Autodesk Inventor part; units mm, degrees
ref_plane "YZ Plane" through (0, 0, 0) normal (1, 0, 0) x (0, 1, 0)
ref_plane "XZ Plane" through (0, 0, 0) normal (0, 1, 0) x (-1, 0, 0)
ref_plane "XY Plane" through (0, 0, 0) normal (0, 0, 1) x (1, 0, 0)
sketch "スケッチ1" plane through (0, 0, 0) normal (0, 0, 1) x (1, 0, 0)
  line L0 (0, 0) -> (85, 0)
  line L1 (85, 0) -> (85, 42)
  line L2 (85, 42) -> (0, 42)
  line L3 (0, 42) -> (0, 0)
  dimension "d0" = 85
  dimension "d1" = 42
extrude "押し出し1" add sketch "スケッチ1" along normal blind 6
sketch "スケッチ2" plane through (0, 0, 0) normal (-1, 0, 0) x (0, 0, 1)
  circle A0 centre (3, 36) radius 1.2
  circle A1 centre (3, 6) radius 1.2
  line L0 (0, 42) -> (6, 42)
  line L1 (0, 0) -> (6, 0)
  dimension "d4" = 2.4
  dimension "d5" = 2.4
  dimension "d6" = 6
  dimension "d7" = 6
extrude "押し出し2" cut sketch "スケッチ2" against normal blind 8
sketch "スケッチ3" plane through (85, 0, 0) normal (1, 0, 0) x (0, 0, -1)
  circle A0 centre (-3, 6) radius 1.2
  circle A1 centre (-3, 6) radius 1.2
  circle A2 centre (-3, 36) radius 1.2
  circle A3 centre (-3, 36) radius 1.2
  point P0 (0, 0)
extrude "押し出し3" cut sketch "スケッチ3" against normal blind 8
sketch "スケッチ4" plane through (0, 0, 6) normal (0, 0, 1) x (1, 0, 0)
  line L0 (0, 0) -> (85, 0)
  line L1 (85, 0) -> (85, 42)
  line L2 (85, 42) -> (0, 42)
  line L3 (0, 42) -> (0, 0)
  line L4 (13.6951, 28.3049) -> (71.3049, 28.3049)
  line L5 (71.3049, 28.3049) -> (71.3049, 13.6951)
  line L6 (71.3049, 13.6951) -> (13.6951, 13.6951)
  line L7 (13.6951, 13.6951) -> (13.6951, 28.3049)
extrude "押し出し4" cut sketch "スケッチ4" against normal blind 10 contours L4 L5 L6 L7
fillet "フィレット1" radius 4 4 edges at (13.6951, 28.3049, 3) (13.6951, 13.6951, 3) (71.3049, 13.6951, 3) (71.3049, 28.3049, 3)
For this review, take the finished solid that the model builds, in its own axes (mm). A direction names the side the tool comes from. Coordinates: 2 decimals unless noted, no trailing zeros. Loops run counter-clockwise (first coordinate to the right, second up) from the corner with the lowest first, then second, coordinate; pieces in that order, holes last. Notation, with made-up numbers: (75.25, 47.5) -> (91.25, 47.5) arc R15 ccw to (91.25, 72.5) -> close; hole circle Ø5 at (45.5, 17.5). An arc over 180 degrees is marked (long way). Return JSON: item names as keys, results as strings. Group by question number.
(1) For pin 1 Ø1.2 at (y, z) = (35.5, 3) entering from -X; pin 2 Ø1.4 at (y, z) = (36, 3) entering from +X, all flat-tipped, find the tip position at first contact; note any pin that passes through.
(2) Tool access review of faces 1 (the flat face through (71.305, 21, 3)), 2 (the cylindrical face through (81.06, 37.19, 3.16)), 3 (the cylindrical face through (3.94, 37.19, 2.84)): name each direction out of +Z, -Z, +X, -X, +Y, -Y from which nothing blocks a thin tool from reaching the whole face with its end or side.
(3) To check wall thickness, follow L1, parallel to Y at x = 81.5, z = 3; L2, parallel to Y at x = 28.5, z = 1.3; L3, parallel to X at y = 36, z = 2.4. State the ranges of each line that lie inside material, in increasing order.
(4) Consider section D-D, the plane y = 36. Give the boundary of the cut face in (x, z), plus the area to 3 significant figures.
(5) Consider section B-B, the plane z = 5.1. Give the boundary of the cut face in (x, y), plus the area to 3 significant figures.
(6) Consider section C-C, the plane y = 21. Give the boundary of the cut face in (x, z).
(7) Mouldability with a two-part tool opening along Z and no side actions: class faces 4 (the flat face through (42, 31, 0)), 5 (the cylindrical face through (81.06, 7.19, 3.16)), 6 (the cylindrical face through (70.102, 27.164, 2.958)) as pulls with the +Z half, pulls with the -Z half, needs draft (parallel to the pull), parting line crosses it, or undercut.
(8) Consider section A-A, the plane x = 66.5. Give the boundary of the cut face in (y, z).
Results below:
{
 "1": {"pin 1": "stops at x = 8", "pin 2": "stops at x = 77"},
 "2": {"face 1": "+Z, -Z", "face 2": "+X", "face 3": "-X"},
 "3": {"L1": "y = 0 to 4.8, 7.2 to 34.8, 37.2 to 42", "L2": "y = 0 to 13.7, 28.3 to 42", "L3": "x = 8 to 77"},
 "4": {"outline": "(0, 0) -> (85, 0) -> (85, 1.8) -> (77, 1.8) -> (77, 4.2) -> (85, 4.2) -> (85, 6) -> (0, 6) -> (0, 4.2) -> (8, 4.2) -> (8, 1.8) -> (0, 1.8) -> close", "area": "472 mm2"},
 "5": {"outline": "(0, 0) -> (85, 0) -> (85, 42) -> (0, 42) -> close; hole (13.7, 17.7) arc R4 ccw to (17.7, 13.7) -> (67.3, 13.7) arc R4 ccw to (71.3, 17.7) -> (71.3, 24.3) arc R4 ccw to (67.3, 28.3) -> (17.7, 28.3) arc R4 ccw to (13.7, 24.3) -> close", "area": "2,740 mm2"},
 "6": {"outline": "(0, 0) -> (13.7, 0) -> (13.7, 6) -> (0, 6) -> close; (71.3, 0) -> (85, 0) -> (85, 6) -> (71.3, 6) -> close"},
 "7": {"face 4": "pulls with the -Z half", "face 5": "undercut", "face 6": "needs draft"},
 "8": {"outline": "(0, 0) -> (13.7, 0) -> (13.7, 6) -> (0, 6) -> close; (28.3, 0) -> (42, 0) -> (42, 6) -> (28.3, 6) -> close"}
}
